Design review of the part built by this model. Coordinates are the model's own, in mm. Face numbers are marked on the shaded views. A direction names the side the tool comes from. Round coordinates to 2 decimals unless told otherwise and drop trailing zeros. Order: outer loops, then holes, each group sorted by start corner. A loop starts at its lowest first (then second) coordinate and runs counter-clockwise, first axis right, second up.
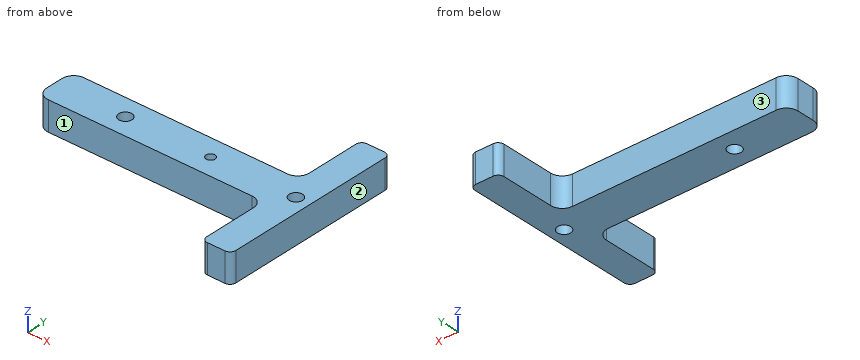
from build123d import *

# Parameters (mm, degrees)
BOSS_EXTRUDE1_DEPTH = 5
SKETCH2_R           = 1.140983763
SKETCH2_R_2         = 1.130194527
CUT_EXTRUDE1_DEPTH  = 32.526020999
SKETCH3_R           = 0.77
CUT_EXTRUDE2_DEPTH  = 3


with BuildPart() as part:
    # Sketch1 → Boss-Extrude1 (new body)
    with BuildSketch(Plane.XY):
        with BuildLine():
            Line((-17.5, 0), (17.5, 0))
            ThreePointArc((17.5, 0), (18.914213562, 0.585786438), (19.5, 2))
            Line((19.5, 2), (19.5, 11.2))
            ThreePointArc((19.5, 11.2), (19.792893219, 11.907106781), (20.5, 12.2))
            Line((20.5, 12.2), (23.5, 12.2))
            ThreePointArc((23.5, 12.2), (24.207106781, 11.907106781), (24.5, 11.2))
            Line((24.5, 11.2), (24.5, -18.2))
            ThreePointArc((24.5, -18.2), (24.207106781, -18.907106781), (23.5, -19.2))
            Line((23.5, -19.2), (20.5, -19.2))
            ThreePointArc((20.5, -19.2), (19.792893219, -18.907106781), (19.5, -18.2))
            Line((19.5, -18.2), (19.5, -9))
            ThreePointArc((19.5, -9), (18.914213562, -7.585786438), (17.5, -7))
            Line((17.5, -7), (-17.5, -7))
            ThreePointArc((-17.5, -7), (-18.914213562, -6.414213562), (-19.5, -5))
            Line((-19.5, -5), (-19.5, -2))
            ThreePointArc((-19.5, -2), (-18.914213562, -0.585786438), (-17.5, 0))
        make_face()
    extrude(amount=BOSS_EXTRUDE1_DEPTH)

    # Sketch2 → Cut-Extrude1 (cut, through all)
    with BuildSketch(Plane.XY.offset(5)):
        with Locations((22, -3.5)):
            Circle(SKETCH2_R)
        with Locations((-7.3, -3.5)):
            Circle(SKETCH2_R_2)
    extrude(amount=-CUT_EXTRUDE1_DEPTH, mode=Mode.SUBTRACT)

    # Sketch3 → Cut-Extrude2 (cut)
    with BuildSketch(Plane.XY.offset(5)):
        with Locations((7.35, -3.5)):
            Circle(SKETCH3_R)
    extrude(amount=-CUT_EXTRUDE2_DEPTH, mode=Mode.SUBTRACT)


solid = part.part
1) Take a section at A-A on x = -7.3. Give the boundary of the cut face in (y, z).
Results:
outline: (-7, 0) - (-4.63, 0) - (-4.63, 5) - (-7, 5) - close; (-2.37, 0) - (0, 0) - (0, 5) - (-2.37, 5) - close
2) To check wall thickness, follow line 1 along Y through (x, z) = (7.35, 4.1); line 2 along Y through (x, z) = (-7.3, 1.8); line 3 along Y through (x, z) = (-16, 1.8). State the ranges of each line that lie inside material, in increasing order.
Results:
line 1: y = -7 to -4.27, -2.73 to 0
line 2: y = -7 to -4.63, -2.37 to 0
line 3: y = -7 to 0
3) Take a section at B-B on y = -3.5. Give the boundary of the cut face in (x, z).
Results:
outline: (-19.5, 0) - (-8.43, 0) - (-8.43, 5) - (-19.5, 5) - close; (-6.17, 0) - (20.86, 0) - (20.86, 5) - (8.12, 5) - (8.12, 2) - (6.58, 2) - (6.58, 5) - (-6.17, 5) - close; (23.14, 0) - (24.5, 0) - (24.5, 5) - (23.14, 5) - close
4) For the marked faces 1, 2 and 3, list the 3-axis set-ups (+Z, -Z, +X, -X, +Y, -Y) from which the entire face can be reached by the end or side of a thin tool; tool diameter is ignored.
Results:
face 1: +Z, -Z, -X, -Y
face 2: +Z, -Z, +X, +Y, -Y
face 3: +Z, -Z, -X, +Y
5) Take a section at D-D on z = 3.6. Give the boundary of the cut face in (x, y).
Results:
outline: (-19.5, -5) arc R2 ccw to (-17.5, -7) - (17.5, -7) arc R2 cw to (19.5, -9) - (19.5, -18.2) arc R1 ccw to (20.5, -19.2) - (23.5, -19.2) arc R1 ccw to (24.5, -18.2) - (24.5, 11.2) arc R1 ccw to (23.5, 12.2) - (20.5, 12.2) arc R1 ccw to (19.5, 11.2) - (19.5, 2) arc R2 cw to (17.5, 0) - (-17.5, 0) arc R2 ccw to (-19.5, -2) - close; hole circle Ø2.26 at (-7.3, -3.5); hole circle Ø1.54 at (7.35, -3.5); hole circle Ø2.28 at (22, -3.5)
6) Take a section at C-C on z = 1. Give the boundary of the cut face in (x, y).
Results:
outline: (-19.5, -5) arc R2 ccw to (-17.5, -7) - (17.5, -7) arc R2 cw to (19.5, -9) - (19.5, -18.2) arc R1 ccw to (20.5, -19.2) - (23.5, -19.2) arc R1 ccw to (24.5, -18.2) - (24.5, 11.2) arc R1 ccw to (23.5, 12.2) - (20.5, 12.2) arc R1 ccw to (19.5, 11.2) - (19.5, 2) arc R2 cw to (17.5, 0) - (-17.5, 0) arc R2 ccw to (-19.5, -2) - close; hole circle Ø2.26 at (-7.3, -3.5); hole circle Ø2.28 at (22, -3.5)
7) Clearance check with flat-ended pins moving along their axes: P1, Ø2.5, axis at x = 1, z = 2, coming from the -Y side; P2, Ø1.5, axis at y = -15, z = 1.5, coming from the -X side; P3, Ø2.5, axis at x = 3, z = 2.5, coming from the +Y side. State where each tip first meets the part, or that it passes through.
Results:
P1: stops at y = -7
P2: stops at x = 19.5
P3: stops at y = 0
